Design review of the part built by this model. Coordinates are the model's own, in mm. A direction names the side the tool comes from. Round coordinates to 2 decimals unless told otherwise and drop trailing zeros. Order: outer loops, then holes, each group sorted by start corner. A loop starts at its lowest first (then second) coordinate and runs counter-clockwise, first axis right, second up. Notation, with made-up numbers: M 9,-1.75 L 55,-1.75 A7 cw 55,7.25 Z; hole C 52.5,76.5 d10. An arc over 180 degrees is marked long. Use a Markdown table: item, result. Add a question column.
(1) Take a section at A-A (x = 50). Write out the cut boundary in (y, z), then the cut area to 3 significant figures.
(2) Take a section at B-B (y = 0). Write out the cut boundary in (x, z), then the cut area to 3 significant figures.
(3) To check wall thickness, follow probe 1 along Y at (x, z) = (0, 2.15); probe 2 along X at (y, z) = (-0.25, 4.2); probe 3 along Y at (x, z) = (35, 0.95). State the ranges of each line that lie inside material, in increasing order. Write a range as from..to.
(4) For pin 1 (1 mm diameter, centred on x = 1, z = 3, fed in from +Y); pin 2 (3 mm diameter, centred on x = 17, y = 3.5, fed in from -Z); pin 3 (1 mm diameter, centred on x = 21, z = 4, fed in from +Y); pin 4 (1 mm diameter, centred on y = 1.5, z = 3, fed in from +X), all flat-tipped, find the tip position at first contact; note any pin that passes through.
(5) Take a section at C-C (z = 1.7). Write out the cut boundary in (x, y).
(6) Machinability: for faces 1 (the face through (51.526, 0.481, 1.479)), 2 (the face through (47, 0, 4)), which of the approach directions +Z, -Z, +X, -X, +Y, -Y give a long, thin tool a straight path to every point of the face, cutting with its end or side? Answer none if there is none.
(7) Take a section at D-D (x = 0). Write out the cut boundary in (y, z), then the cut area to 3 significant figures.
```python
from build123d import *

# Parameters (mm, degrees)
SKETCH1_R           = 1.6
BOSS_EXTRUDE1_DEPTH = 5
SKETCH2_R           = 3
CUT_EXTRUDE1_DEPTH  = 2
BOSS_EXTRUDE2_START = -5
SKETCH3_R           = 7
SKETCH3_R_2         = 4.7
BOSS_EXTRUDE2_DEPTH = 5
FILLET1_R           = 1


with BuildPart() as part:
    # Sketch1 → Boss-Extrude1 (new body)
    with BuildSketch(Plane.XY):
        with BuildLine():
            ThreePointArc((0, 4.7), (-4.7, 0), (0, -4.7))
            Line((0, -4.7), (50, -4.7))
            ThreePointArc((50, -4.7), (54.7, 0), (50, 4.7))
            Line((50, 4.7), (0, 4.7))
        make_face()
        Circle(SKETCH1_R, mode=Mode.SUBTRACT)
        with Locations((50, 0)):
            Circle(SKETCH1_R, mode=Mode.SUBTRACT)
    extrude(amount=BOSS_EXTRUDE1_DEPTH)

    # Sketch2 → Cut-Extrude1 (cut)
    with BuildSketch(Plane.XY.offset(5)):
        with Locations((50, 0)):
            Circle(SKETCH2_R)
    extrude(amount=-CUT_EXTRUDE1_DEPTH, mode=Mode.SUBTRACT)

    # Sketch3 → Boss-Extrude2 (add)
    # profile 1 of 2: a face of its own
    with BuildSketch(Plane.XY.offset(5).offset(BOSS_EXTRUDE2_START)):
        with Locations((50, 0)):
            Circle(SKETCH3_R)
        with Locations((50, 0)):
            Circle(SKETCH3_R_2, mode=Mode.SUBTRACT)
    # profile 2 of 2: a face of its own
    with BuildSketch(Plane.XY.offset(5).offset(BOSS_EXTRUDE2_START)):
        Circle(SKETCH3_R)
        Circle(SKETCH3_R_2, mode=Mode.SUBTRACT)
    extrude(amount=BOSS_EXTRUDE2_DEPTH)

    # Fillet1
    fillet1_edges = [part.edges().sort_by_distance(p)[0] for p in [
        (57, 0, 5),
        (57, 0, 0),
    ]]
    fillet(fillet1_edges, radius=FILLET1_R)


solid = part.part
```
Verdict:
| question | item | result |
|---|---|---|
| 1 | outline | M -7,1 A1 ccw -6,0 L -1.6,0 L -1.6,3 L -3,3 L -3,5 L -6,5 A1 ccw -7,4 Z; M 1.6,0 L 6,0 A1 ccw 7,1 L 7,4 A1 ccw 6,5 L 3,5 L 3,3 L 1.6,3 Z |
| 1 | area | 47.5 mm^2 |
| 2 | outline | M -7,0 L -1.6,0 L -1.6,5 L -7,5 Z; M 1.6,0 L 48.4,0 L 48.4,3 L 47,3 L 47,5 L 1.6,5 Z; M 51.6,0 L 56,0 A1 ccw 57,1 L 57,4 A1 ccw 56,5 L 53,5 L 53,3 L 51.6,3 Z |
| 2 | area | 282 mm^2 |
| 3 | probe 1 | y = -7..-1.6, 1.6..7 |
| 3 | probe 2 | x = -7..-1.58, 1.58..47.01, 52.99..56.98 |
| 3 | probe 3 | y = -4.7..4.7 |
| 4 | pin 1 | stops at y = 6.98 |
| 4 | pin 2 | stops at z = 0 |
| 4 | pin 3 | stops at y = 4.7 |
| 4 | pin 4 | stops at x = 56.93 |
| 5 | outline | M 5.19,-4.7 L 44.81,-4.7 A7 ccw long 44.81,4.7 L 5.19,4.7 A7 ccw long Z; hole C 0,0 d3.2; hole C 50,0 d3.2 |
| 6 | face 1 | +Z, -Z |
| 6 | face 2 | +Z |
| 7 | outline | M -7,0 L -1.6,0 L -1.6,5 L -7,5 Z; M 1.6,0 L 7,0 L 7,5 L 1.6,5 Z |
| 7 | area | 54.0 mm^2 |
